Could you check a few things on this model? Use its own coordinates, in mm. Coordinates: 2 decimals unless noted, no trailing zeros. Write each loop counter-clockwise with the first axis right and the second up, starting at its lowest first coordinate (ties: lowest second). Pieces come first, ordered by that corner, then holes. Notation, with made-up numbers: (36.5, 13.5) - (41.5, 13.5) arc R23 cw to (41.5, 22.5) - close; hole circle Ø11 at (-6.75, 80.5). An arc over 180 degrees is marked (long way). Answer as a JSON object with one key per item and string values. Group by question number.
1) If we section it at A-A (x = 100): Write out the boundary of the cut face in (y, z), plus the area to 3 significant figures.
2) Will this pin go through, and if not, where does the flat tip stop? pin 1 Ø9 at (x, z) = (100, 7.5) entering from -Y.
3) If we section it at B-B (z = 8.5): Write out the boundary of the cut face in (x, y), plus the area to 3 significant figures.
4) Please list where these lines run through material, in increasing order: line 1 along X through (y, z) = (3.75, 4); line 2 along X through (y, z) = (23, 7.5); line 3 along X through (y, z) = (11.5, 7.5).
5) If we section it at C-C (y = 9.5): Write out the boundary of the cut face in (x, z), plus the area to 3 significant figures.
6) We'd pull the mould along Z, two halves only. Please class faces 1 (the flat face through (-2, 0, 7)), 2 (the cylindrical face through (101.5, 14.79, 2.73)), 3 (the flat face through (2, 5, 0)), 4 (the cylindrical face through (-104.88, 14.79, 8.58)): released by +Z, released by -Z, zero draft, split by the parting line, or undercut.
```python
from build123d import *

# Parameters (mm, degrees)
RESSALTO_EXTRUS_O1_DEPTH = 15
CORTE_EXTRUS_O1_DEPTH    = 15
ESBO_O10_R               = 5
CORTE_EXTRUS_O9_DEPTH    = 79


with BuildPart() as part:
    # Esboço1 → Ressalto-extrusão1 (new body)
    with BuildSketch(Plane.XY):
        Polygon((100, 0), (-100, 0), (-120, 0), (-120, 30), (-100, 30), (100, 30), (120, 30), (120, 0), align=None)
    extrude(amount=RESSALTO_EXTRUS_O1_DEPTH)

    # Esboço2 → Corte-extrusão1 (cut)
    with BuildSketch(Plane.XY.offset(15)):
        with BuildLine():
            ThreePointArc((7.5, 15), (5.303300859, 20.303300859), (0, 22.5))
            Line((0, 22.5), (0, 7.5))
            ThreePointArc((0, 7.5), (5.303300859, 9.696699141), (7.5, 15))
        make_face()
        with BuildLine():
            Line((0, 7.5), (0, 22.5))
            ThreePointArc((0, 22.5), (-7.5, 15), (0, 7.5))
        make_face()
    extrude(amount=-CORTE_EXTRUS_O1_DEPTH, mode=Mode.SUBTRACT)

    # Esboço10 → Corte-extrusão9 (cut)
    with BuildSketch(Plane(origin=(0, 0, 0), x_dir=(-1, 0, 0), z_dir=(0, -1, 0))):
        with Locations(Location((100, -7.5, 0), (0, 0, 90))):
            Circle(ESBO_O10_R)
        with Locations(Location((-100, -7.5, 0), (0, 0, 90))):
            Circle(ESBO_O10_R)
    extrude(amount=-CORTE_EXTRUS_O9_DEPTH, mode=Mode.SUBTRACT)


solid = part.part
```
Here are the results:
{
 "1": {"outline": "(0, 0) - (30, 0) - (30, 2.5) - (0, 2.5) - close; (0, 12.5) - (30, 12.5) - (30, 15) - (0, 15) - close", "area": "150 mm²"},
 "2": {"pin 1": "passes through"},
 "3": {"outline": "(-120, 0) - (-104.9, 0) - (-104.9, 30) - (-120, 30) - close; (-95.1, 0) - (95.1, 0) - (95.1, 30) - (-95.1, 30) - close; (104.9, 0) - (120, 0) - (120, 30) - (104.9, 30) - close; hole circle Ø15 at (0, 15)", "area": "6,440 mm²"},
 "4": {"line 1": "x = -120 to -103.57, -96.43 to 96.43, 103.57 to 120", "line 2": "x = -120 to -105, -95 to 95, 105 to 120", "line 3": "x = -120 to -105, -95 to -6.63, 6.63 to 95, 105 to 120"},
 "5": {"outline": "(-120, 0) - (-5.1, 0) - (-5.1, 15) - (-120, 15) - close; (5.1, 0) - (120, 0) - (120, 15) - (5.1, 15) - close; hole circle Ø10 at (-100, 7.5); hole circle Ø10 at (100, 7.5)", "area": "3,290 mm²"},
 "6": {"face 1": "zero draft", "face 2": "undercut", "face 3": "released by -Z", "face 4": "undercut"}
}
